The listing builds one solid part. Answer for the finished solid, in the listing's coordinates (mm). A direction names the side the tool comes from. Coordinates: 2 decimals unless noted, no trailing zeros. Loops run counter-clockwise (first coordinate to the right, second up) from the corner with the lowest first, then second, coordinate; pieces in that order, holes last. Notation, with made-up numbers: (-39, 28.25) - (-24, 28.25) arc R17 cw to (-24, 44.25) - close; hole circle Ø8 at (54.5, 74). An arc over 180 degrees is marked (long way). Write each question's results on one line, items separated by ' | '. Start each with the question number.
(1) For faces 4 (the flat face through (25, -14, 22)), 5 (the flat face through (20, -10.5, 25)), 6 (the flat face through (-12, -12, 22)), 7 (the flat face through (23, -9.302, 25)), 8 (the flat face through (0, 1, 0)), determine the directions among +Z, -Z, +X, -X, +Y, -Y from which every point of the face is accessible in a straight line to the end or side of a thin tool.
(2) Find section A-A on x = -20. Determine the outline of the cut face in (y, z).
(3) Find section C-C on x = -11.5. Determine the outline of the cut face in (y, z).
(4) Find section D-D on y = 23.5. Determine the outline of the cut face in (x, z), then the cut area to 3 significant figures.
(5) Determine the mould class of faces 1 (the flat face through (0, 1, 45)), 2 (the flat face through (-13, 13, 22)), 3 (the flat face through (0, 30, 22)) for opening direction Y: released by +Y, released by -Y, zero draft, split by the parting line, or undercut.
(6) Consider line 1 (Y direction, x = -6.5, z = 24); line 2 (Y direction, x = -5, z = 5); line 3 (X direction, y = -5, z = 13). Determine where each line is inside the solid, lowest interval first. Write a range as from..to.
(7) Given pin 1 Ø1.5 at (x, z) = (23, 28) entering from -Y; pin 2 Ø3 at (x, z) = (-13.5, 36) entering from +Y; pin 3 Ø0.9 at (x, z) = (23, 23) entering from +Y, each flat-ended and moving along its own axis, determine where each tip first touches the part or whether it passes through.
(8) Find section B-B on z = 23. Determine the outline of the cut face in (x, y), then the cut area to 3 significant figures.
from build123d import *

# Parameters (mm, degrees)
PAD_DEPTH    = 45
POCKET_DEPTH = 40


with BuildPart() as part:
    # Sketch → Pad (new body)
    with BuildSketch(Plane.XY):
        Polygon((-25, 25), (0, 0), (-25, -25), (-25, -40), (25, -20), (25, 20), (-25, 40), align=None)
    extrude(amount=PAD_DEPTH)

    # Sketch001 (on Face9 of Pad) → Pocket (cut)
    with BuildSketch(Plane.XY.offset(45)):
        Polygon((25, 9.302202), (22, 9.302202), (22, 10.5), (17.5, 10.5), (17.5, -10.5), (22, -10.5), (22, -9.302202), (25, -9.302202), align=None)
    extrude(amount=-POCKET_DEPTH, mode=Mode.SUBTRACT)


solid = part.part
Values:
1) face 4: +Z, -Z, +X, +Y, -Y | face 5: +Z | face 6: +Z, -Z, -X | face 7: +Z, +X | face 8: -Z, +X, -X, +Y, -Y
2) outline: (-38, 0) - (-20, 0) - (-20, 45) - (-38, 45) - close; (20, 0) - (38, 0) - (38, 45) - (20, 45) - close
3) outline: (-34.6, 0) - (-11.5, 0) - (-11.5, 45) - (-34.6, 45) - close; (11.5, 0) - (34.6, 0) - (34.6, 45) - (11.5, 45) - close
4) outline: (-23.5, 0) - (16.25, 0) - (16.25, 45) - (-23.5, 45) - close | area: 1,790 mm²
5) face 1: zero draft | face 2: undercut | face 3: released by +Y
6) line 1: y = -32.6..-6.5, 6.5..32.6 | line 2: y = -32..-5, 5..32 | line 3: x = -5..17.5
7) pin 1: stops at y = -21.1 | pin 2: stops at y = 36 | pin 3: stops at y = 20.98
8) outline: (-25, -40) - (25, -20) - (25, -9.3) - (22, -9.3) - (22, -10.5) - (17.5, -10.5) - (17.5, 10.5) - (22, 10.5) - (22, 9.3) - (25, 9.3) - (25, 20) - (-25, 40) - (-25, 25) - (0, 0) - (-25, -25) - close | area: 2,220 mm²
